```python
from build123d import *

# Parameters (mm, degrees)
F1_DEPTH = 30
F3_DEPTH = 370


with BuildPart() as f1:
    # F0 (on Top) → F1 (new body)
    with BuildSketch(Plane.XY):
        with BuildLine():
            Line((157.539008, 220.72852), (-202.460992, 220.72852))
            ThreePointArc((-202.460992, 220.72852), (-216.603128, 214.870655), (-222.460992, 200.72852))
            Line((-222.460992, 200.72852), (-222.460992, -159.27148))
            ThreePointArc((-222.460992, -159.27148), (-216.603128, -173.413616), (-202.460992, -179.27148))
            Line((-202.460992, -179.27148), (157.539008, -179.27148))
            ThreePointArc((157.539008, -179.27148), (171.681143, -173.413616), (177.539008, -159.27148))
            Line((177.539008, -159.27148), (177.539008, 200.72852))
            ThreePointArc((177.539008, 200.72852), (171.681143, 214.870655), (157.539008, 220.72852))
        make_face()
    extrude(amount=F1_DEPTH)

    # F2 (on face) → F3 (join)
    with BuildSketch(Plane.XY.offset(30)):
        with BuildLine():
            Line((-152.460992, 180.72852), (-172.460992, 180.72852))
            ThreePointArc((-172.460992, 180.72852), (-179.53206, 177.799588), (-182.460992, 170.72852))
            Line((-182.460992, 170.72852), (-182.460992, 150.72852))
            ThreePointArc((-182.460992, 150.72852), (-179.53206, 143.657452), (-172.460992, 140.72852))
            Line((-172.460992, 140.72852), (-152.460992, 140.72852))
            ThreePointArc((-152.460992, 140.72852), (-145.389924, 143.657452), (-142.460992, 150.72852))
            Line((-142.460992, 150.72852), (-142.460992, 170.72852))
            ThreePointArc((-142.460992, 170.72852), (-145.389924, 177.799588), (-152.460992, 180.72852))
        make_face()
        with BuildLine():
            Line((127.539008, 180.72852), (107.539008, 180.72852))
            ThreePointArc((107.539008, 180.72852), (100.46794, 177.799588), (97.539008, 170.72852))
            Line((97.539008, 170.72852), (97.539008, 150.72852))
            ThreePointArc((97.539008, 150.72852), (100.46794, 143.657452), (107.539008, 140.72852))
            Line((107.539008, 140.72852), (127.539008, 140.72852))
            ThreePointArc((127.539008, 140.72852), (134.610076, 143.657452), (137.539008, 150.72852))
            Line((137.539008, 150.72852), (137.539008, 170.72852))
            ThreePointArc((137.539008, 170.72852), (134.610076, 177.799588), (127.539008, 180.72852))
        make_face()
        with BuildLine():
            Line((127.539008, -99.27148), (107.539008, -99.27148))
            ThreePointArc((107.539008, -99.27148), (100.46794, -102.200412), (97.539008, -109.27148))
            Line((97.539008, -109.27148), (97.539008, -129.27148))
            ThreePointArc((97.539008, -129.27148), (100.46794, -136.342548), (107.539008, -139.27148))
            Line((107.539008, -139.27148), (127.539008, -139.27148))
            ThreePointArc((127.539008, -139.27148), (134.610076, -136.342548), (137.539008, -129.27148))
            Line((137.539008, -129.27148), (137.539008, -109.27148))
            ThreePointArc((137.539008, -109.27148), (134.610076, -102.200412), (127.539008, -99.27148))
        make_face()
        with BuildLine():
            Line((-152.460992, -99.27148), (-172.460992, -99.27148))
            ThreePointArc((-172.460992, -99.27148), (-179.53206, -102.200412), (-182.460992, -109.27148))
            Line((-182.460992, -109.27148), (-182.460992, -129.27148))
            ThreePointArc((-182.460992, -129.27148), (-179.53206, -136.342548), (-172.460992, -139.27148))
            Line((-172.460992, -139.27148), (-152.460992, -139.27148))
            ThreePointArc((-152.460992, -139.27148), (-145.389924, -136.342548), (-142.460992, -129.27148))
            Line((-142.460992, -129.27148), (-142.460992, -109.27148))
            ThreePointArc((-142.460992, -109.27148), (-145.389924, -102.200412), (-152.460992, -99.27148))
        make_face()
    extrude(amount=F3_DEPTH)


solid = f1.part
```
Geometry check sheet. Reference: the model listing, model coordinates, mm. A direction names the side the tool comes from. Round coordinates to 2 decimals unless told otherwise and drop trailing zeros. Loops run counter-clockwise (first coordinate to the right, second up) from the corner with the lowest first, then second, coordinate; pieces in that order, holes last. Notation, with made-up numbers: M 51,75 L 71,75 A26 ccw 71,89 Z; hole C 41.5,57.5 d4. An arc over 180 degrees is marked long. Return JSON: item names as keys, results as strings. Group by question number.
(1) Go/stop test with flat-tipped pins: pin 1 (1.5 mm diameter, centred on x = -142, y = 102.5, fed in from -Z); pin 2 (8 mm diameter, centred on x = 3, y = 114, fed in from +Z); pin 3 (16 mm diameter, centred on x = 114, z = 298, fed in from +Y); pin 4 (1.5 mm diameter, centred on x = -142.5, z = 168.5, fed in from -Y). Record where each tip stops, or that it passes through.
(2) Set-up check for faces 1 (the face through (-162, 180.729, 212)), 2 (the face through (-182.461, 161, 212)), 3 (the face through (-163, 140.729, 212)), 4 (the face through (97.539, -119, 212)): record each of +Z, -Z, +X, -X, +Y, -Y from which the full face is reachable in a straight line by a thin tool's end or side.
(3) Section check B-B, the plane y = -38. Enter the section's corners in (x, z), and give its area (3 significant figures).
(4) Section check C-C, the plane x = 43. Enter the section's corners in (y, z), and give its area (3 significant figures).
(5) Mould release check, pull along Y, two halves, no side actions. Record for faces 5 (the face through (-20, 220.729, 15)), 6 (the face through (-142.461, 161, 212)), 7 (the face through (-162, -99.271, 212)), 8 (the face through (-25, -179.271, 15)): pulls with the +Y half, pulls with the -Y half, needs draft (parallel to the pull), parting line crosses it, or undercut.
(6) Section check A-A, the plane z = 168. Give the number of separate pieces and of enclosed holes in the cut face, and give its area (3 significant figures).
(7) Scan lines: line 1 along Y through (x, z) = (129, 257); line 2 along Y through (x, z) = (109.5, 287.5); line 3 along X through (y, z) = (-123, 169.5). Record each from-to range of solid material in increasing order. Write a range as [from, to].
Data:
{
 "1": {"pin 1": "z = 0", "pin 2": "z = 30", "pin 3": "y = 180.73", "pin 4": "y = -133.16"},
 "2": {"face 1": "+Z, +X, -X, +Y", "face 2": "+Z, -X, +Y, -Y", "face 3": "+Z, +X, -X", "face 4": "+Z, +Y, -Y"},
 "3": {"outline": "M -222.46,0 L 177.54,0 L 177.54,30 L -222.46,30 Z", "area": "12,000 mm²"},
 "4": {"outline": "M -179.27,0 L 220.73,0 L 220.73,30 L -179.27,30 Z", "area": "12,000 mm²"},
 "5": {"face 5": "pulls with the +Y half", "face 6": "needs draft", "face 7": "undercut", "face 8": "pulls with the -Y half"},
 "6": {"separate pieces": "4", "enclosed holes": "0", "area": "6,060 mm²"},
 "7": {"line 1": "[-139.16, -99.38], [140.84, 180.62]", "line 2": "[-139.27, -99.27], [140.73, 180.73]", "line 3": "[-182.46, -142.46], [97.54, 137.54]"}
}
